Could you check a few things on this drawing? It's one solid part, dimensions in mm from its lowest x, y, z. Coordinates: 2 decimals unless noted, no trailing zeros. Order: outer loops, then holes, each group sorted by start corner. A loop starts at its lowest first (then second) coordinate and runs counter-clockwise, first axis right, second up. Notation, with made-up numbers: (5.5, 33) - (50.5, 33) arc R19 ccw to (50.5, 52) - close; hole circle Ø3 at (-31.5, -20). An arc over 180 degrees is marked (long way). Answer in a Markdown table with one row per item. Add a question column.
Item 1: I want a section at A-A (z = 25). Please give me the cut outline in (x, y).
Item 2: I want a section at C-C (y = 2.7). Count the separate pieces of the cut face and the enclosed holes in it, plus the area to 3 significant figures.
Item 3: I want a section at D-D (x = 36.5). Please give me the cut outline in (y, z).
Item 4: Will these pins go through, and if not, where does the flat tip stop? pin 1 Ø2 at (y, z) = (2.5, 53.5) entering from +X; pin 2 Ø1.5 at (y, z) = (1.5, 34) entering from -X; pin 3 Ø1 at (y, z) = (1, 9) entering from -X (1 decimal).
Item 5: I want a section at B-B (x = 25). Please give me the cut outline in (y, z).
Item 6: If I drill on line 1 along X through (y, z) = (1.9, 13.5); line 2 along X through (y, z) = (1, 27); line 3 along X through (y, z) = (2.35, 41.5), over which ranges is the centre line in solid material (lowest first)? Write a range as from..to.
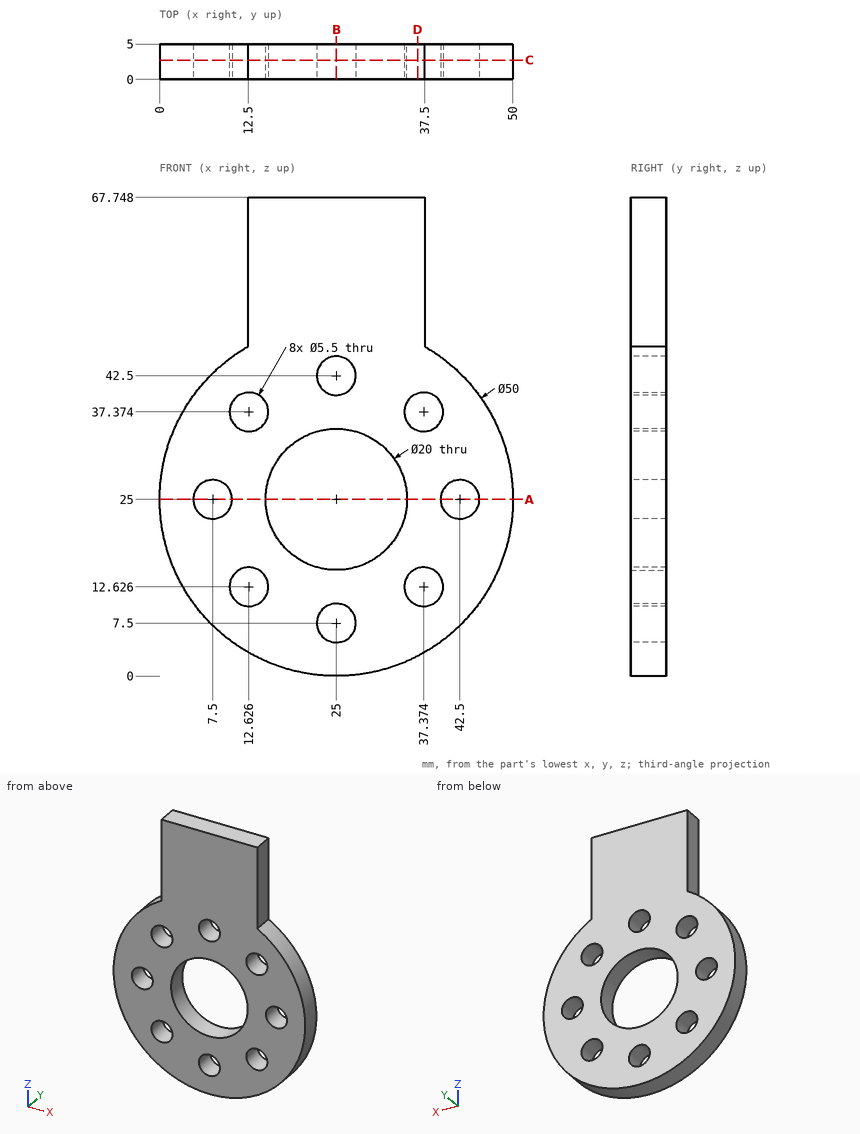
Values follow:
| question | item | result |
|---|---|---|
| 1 | outline | (0, 0) - (4.75, 0) - (4.75, 5) - (0, 5) - close; (10.25, 0) - (15, 0) - (15, 5) - (10.25, 5) - close; (35, 0) - (39.75, 0) - (39.75, 5) - (35, 5) - close; (45.25, 0) - (50, 0) - (50, 5) - (45.25, 5) - close |
| 2 | separate pieces | 1 |
| 2 | enclosed holes | 9 |
| 2 | area | 1,930 mm^2 |
| 3 | outline | (0, 2.8) - (5, 2.8) - (5, 10.02) - (0, 10.02) - close; (0, 15.23) - (5, 15.23) - (5, 34.77) - (0, 34.77) - close; (0, 39.98) - (5, 39.98) - (5, 67.75) - (0, 67.75) - close |
| 4 | pin 1 | stops at x = 37.5 |
| 4 | pin 2 | stops at x = 1.4 |
| 4 | pin 3 | stops at x = 5.4 |
| 5 | outline | (0, 0) - (5, 0) - (5, 4.75) - (0, 4.75) - close; (0, 10.25) - (5, 10.25) - (5, 15) - (0, 15) - close; (0, 35) - (5, 35) - (5, 39.75) - (0, 39.75) - close; (0, 45.25) - (5, 45.25) - (5, 67.75) - (0, 67.75) - close |
| 6 | line 1 | x = 2.8..10.02, 15.23..34.77, 39.98..47.2 |
| 6 | line 2 | x = 0.08..5.61, 9.39..15.2, 34.8..40.61, 44.39..49.92 |
| 6 | line 3 | x = 6.22..22.44, 27.56..43.78 |
